Could you check a few things on this drawing? It's one solid part, dimensions in mm from its lowest x, y, z. A direction names the side the tool comes from. Round coordinates to 2 decimals unless told otherwise and drop trailing zeros. Order: outer loops, then holes, each group sorted by start corner. A loop starts at its lowest first (then second) coordinate and runs counter-clockwise, first axis right, second up. Notation, with made-up numbers: (22.25, -26) -> (75.25, -26) arc R17 cw to (75.25, -6) -> close; hole circle Ø8 at (70, -7.5). An arc over 180 degrees is marked (long way). Use a Markdown table: item, result. Add a question column.
(1) I want a section at D-D, the plane z = 21.5. Please give me the cut outline in (x, y).
(2) Thinking about a two-plate mould opening in Y: for the marked faces 3, 4 and 5, which applies, pulls with the +Y half, pulls with the -Y half, needs draft (parallel to the pull), parting line crosses it, or undercut?
(3) I want a section at B-B, the plane z = 4.5. Please give me the cut outline in (x, y).
(4) On a 3-axis mill with a long thin cutter (end or side, diameter ignored), from which of +Z, -Z, +X, -X, +Y, -Y can I reach the whole of each face in a straight line? I mean the marked faces 1 and 2. Say none if no direction works.
(5) I'm going to push flat-ended pins straight in: P1, Ø8, axis at x = 11.5, z = 15, coming from the -Y side; P2, Ø14, axis at x = 25.5, y = 14.5, coming from the +Z side; P3, Ø0.9, axis at x = 0.5, y = 19, coming from the +Z side. Where does each tip first touch, or does it pass through?
(6) If I drill on probe 1 along Y at (x, z) = (3, 10.75); probe 2 along X at (y, z) = (3, 28.75); probe 3 along Z at (x, y) = (40, 9), over which ranges is the centre line in solid material (lowest first)?
(7) I want a section at C-C, the plane y = 3. Please give me the cut outline in (x, z).
(8) I want a section at A-A, the plane x = 10. Please give me the cut outline in (y, z).
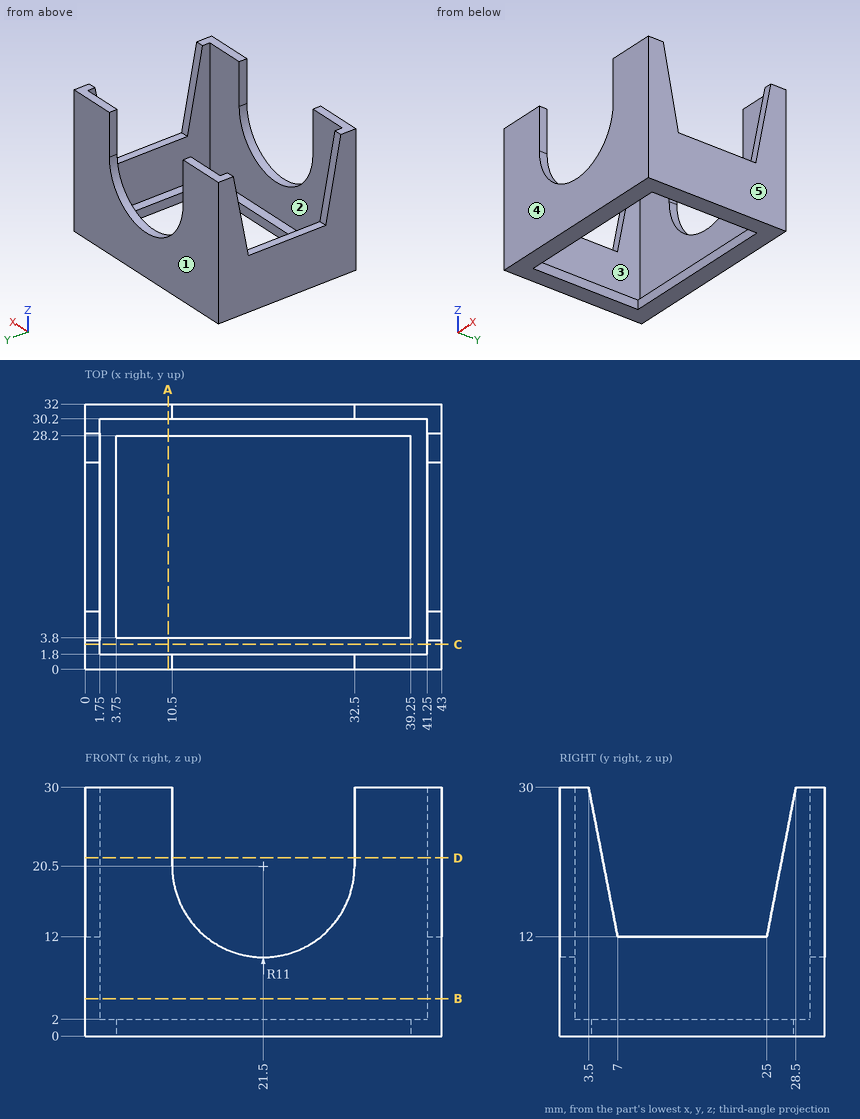
Taken from the geometry:
| question | item | result |
|---|---|---|
| 1 | outline | (0, 0) -> (10.5, 0) -> (10.5, 1.8) -> (1.75, 1.8) -> (1.75, 5.15) -> (0, 5.15) -> close; (0, 26.85) -> (1.75, 26.85) -> (1.75, 30.2) -> (10.5, 30.2) -> (10.5, 32) -> (0, 32) -> close; (32.5, 0) -> (43, 0) -> (43, 5.15) -> (41.25, 5.15) -> (41.25, 1.8) -> (32.5, 1.8) -> close; (32.5, 30.2) -> (41.25, 30.2) -> (41.25, 26.85) -> (43, 26.85) -> (43, 32) -> (32.5, 32) -> close |
| 2 | face 3 | undercut |
| 2 | face 4 | pulls with the -Y half |
| 2 | face 5 | needs draft |
| 3 | outline | (0, 0) -> (43, 0) -> (43, 32) -> (0, 32) -> close; hole (1.75, 1.8) -> (41.25, 1.8) -> (41.25, 30.2) -> (1.75, 30.2) -> close |
| 4 | face 1 | +Z, -Z, +X, -X, +Y |
| 4 | face 2 | +Z |
| 5 | P1 | stops at y = 0 |
| 5 | P2 | passes through |
| 5 | P3 | stops at z = 12 |
| 6 | probe 1 | y = 0 to 1.8, 30.2 to 32 |
| 6 | probe 2 | x = 0 to 1.75, 41.25 to 43 |
| 6 | probe 3 | z = 0 to 2 |
| 7 | outline | (0, 0) -> (43, 0) -> (43, 30) -> (41.25, 30) -> (41.25, 2) -> (1.75, 2) -> (1.75, 30) -> (0, 30) -> close |
| 8 | outline | (0, 0) -> (3.8, 0) -> (3.8, 2) -> (1.8, 2) -> (1.8, 30) -> (0, 30) -> close; (28.2, 0) -> (32, 0) -> (32, 30) -> (30.2, 30) -> (30.2, 2) -> (28.2, 2) -> close |
